Here's the drawing with two shaded views (mm, measured from the low corner). I have some questions. A direction names the side the tool comes from. Round coordinates to 2 decimals unless told otherwise and drop trailing zeros. Loops run counter-clockwise (first coordinate to the right, second up) from the corner with the lowest first, then second, coordinate; pieces in that order, holes last.
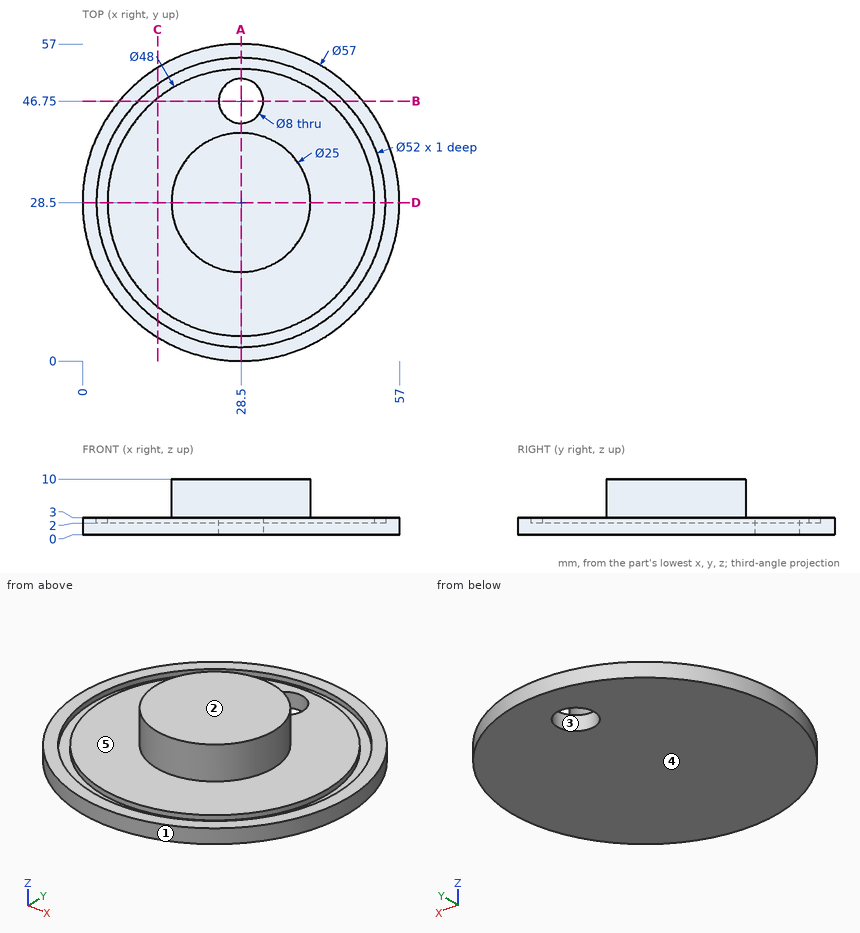
Item 1: If we section it at B-B, the plane y = 46.75: Please give me the cut outline in (x, z).
Results list:
outline: (6.61, 0) - (24.5, 0) - (24.5, 3) - (12.91, 3) - (12.91, 2) - (9.98, 2) - (9.98, 3) - (6.61, 3) - close; (32.5, 0) - (50.39, 0) - (50.39, 3) - (47.02, 3) - (47.02, 2) - (44.09, 2) - (44.09, 3) - (32.5, 3) - close
Item 2: Will these pins go through, and if not, where does the flat tip stop? pin 1 (5 mm diameter, centred on x = 51, z = 2.5, fed in from -Y); pin 2 (6.5 mm diameter, centred on x = 28.5, y = 46.75, fed in from -Z); pin 3 (1.5 mm diameter, centred on x = 32, y = 15.5, fed in from +Z); pin 4 (1.5 mm diameter, centred on y = 39, z = 2.5, fed in from +X).
Results list:
pin 1: stops at y = 8.2
pin 2: passes through
pin 3: stops at z = 3
pin 4: stops at x = 55.28
Item 3: We'd pull the mould along Y, two halves only. Please class the marked faces 1, 2 and 3: released by +Y, released by -Y, zero draft, split by the parting line, or undercut.
Results list:
face 1: split by the parting line
face 2: zero draft
face 3: undercut
Item 4: If I drill on line 1 along Y through (x, z) = (28.5, 2.65); line 2 along X through (y, z) = (11.5, 2.5); line 3 along Y through (x, z) = (39.5, 2.5), over which ranges is the centre line in solid material (lowest first)?
Results list:
line 1: y = 0 to 2.5, 4.5 to 42.75, 50.75 to 52.5, 54.5 to 57
line 2: x = 5.63 to 8.83, 11.56 to 45.44, 48.17 to 51.37
line 3: y = 2.21 to 4.94, 7.17 to 49.83, 52.06 to 54.79
Item 5: If we section it at C-C, the plane x = 13.5: Please give me the cut outline in (y, z) (3 decimals).
Results list:
outline: (4.267, 0) - (52.733, 0) - (52.733, 3) - (49.737, 3) - (49.737, 2) - (47.235, 2) - (47.235, 3) - (9.765, 3) - (9.765, 2) - (7.263, 2) - (7.263, 3) - (4.267, 3) - close
Item 6: For the marked faces 4 and 5, which set-ups out of +Z, -Z, +X, -X, +Y, -Y let a thin tool reach every point of the face, with its end or its side?
Results list:
face 4: -Z, +X, -X, +Y, -Y
face 5: +Z
Item 7: If we section it at A-A, the plane x = 28.5: Please give me the cut outline in (y, z).
Results list:
outline: (0, 0) - (42.75, 0) - (42.75, 3) - (41, 3) - (41, 10) - (16, 10) - (16, 3) - (4.5, 3) - (4.5, 2) - (2.5, 2) - (2.5, 3) - (0, 3) - close; (50.75, 0) - (57, 0) - (57, 3) - (54.5, 3) - (54.5, 2) - (52.5, 2) - (52.5, 3) - (50.75, 3) - close
Item 8: If we section it at D-D, the plane y = 28.5: Please give me the cut outline in (x, z).
Results list:
outline: (0, 0) - (57, 0) - (57, 3) - (54.5, 3) - (54.5, 2) - (52.5, 2) - (52.5, 3) - (41, 3) - (41, 10) - (16, 10) - (16, 3) - (4.5, 3) - (4.5, 2) - (2.5, 2) - (2.5, 3) - (0, 3) - close
